The model under review builds one solid part; all positions refer to its coordinate system, in mm. A direction names the side the tool comes from. Give positions to 0.01 mm unless a question says otherwise; leave off trailing zeros. Order: outer loops, then holes, each group sorted by start corner. A loop starts at its lowest first (then second) coordinate and runs counter-clockwise, first axis right, second up. Notation, with made-up numbers: M 40,23 L 70,23 A19 cw 70,50 Z; hole C -32,22 d1. An arc over 180 degrees is marked long. One line per question, with ' | ' between items. Start each with the question number.
1. We need section C-C on z = 2.5. Write out the cut boundary in (x, y), then the cut area to 3 significant figures.
2. The part is to be moulded in two halves that separate along X. For faces 1 (the face through (-24.927, -8, -1)), 2 (the face through (-12.3, -0.6, 6.5)), 3 (the face through (-24.4, -6.1, 7.404)), say which applies: +X half, -X half, draft (parallel to the pull), parting line (faces both ways), or undercut.
3. Insertion check: P1, Ø8.5, axis at x = -15.4, z = -6.46, coming from the +Y side; P2, Ø5, axis at y = -6, z = 2, coming from the -X side; P3, Ø8, axis at x = 8.5, z = -2, coming from the -Y side; P4, Ø1.1, axis at x = 25.5, y = -8, coming from the -Z side. Each pin has a flat end and moves straight along its axis. Give the tip position at first contact, or say it passes through.
4. Wall thickness on L1, parallel to Z at x = 0, y = -0.95; L2, parallel to X at y = -9, z = -9; L3, parallel to X at y = -0.25, z = -4.75 (3 decimals): over which ranges is each line inside the solid? List them lowest first.
5. For faces 4 (the face through (24.807, -6, -3)), 5 (the face through (25.848, -5, -3)), list the 3-axis set-ups (+Z, -Z, +X, -X, +Y, -Y) from which the entire face can be reached by the end or side of a thin tool; tool diameter is ignored.
6. We need section A-A on y = -2. Write out the cut boundary in (x, z), then the cut area to 3 significant figures.
7. We need section B-B on x = 0. Write out the cut boundary in (y, z).
8. We need section D-D on y = -6.5. Write out the cut boundary in (x, z).
```python
from build123d import *

# Parameters (mm, degrees)
F0_W     = 50.8
F0_H     = 25.4
F1_DEPTH = 1.27
F3_D     = 6.35
F4_R     = 5.08
F5_W     = 1.0414
F5_H     = 16.51
F6_DEPTH = 10.9728
F7_DEPTH = 0.254
F9_D     = 3.81


with BuildPart() as f1:
    # F0 (on Front) → F1 (new body)
    with BuildSketch(Plane.XZ):
        with Locations((0.432136, -0.480445)):
            Rectangle(F0_W, F0_H)
    extrude(amount=F1_DEPTH)

    # F3 (through all)
    with Locations(Plane.XZ.offset(1.27)):
        with Locations((0, -6.53336), (16.458306, 6.398361), (0, 6.395109), (16.458306, -6.737123), (-15.397238, -6.455945), (-15.474654, 6.395109)):
            Hole(F3_D / 2)

    # F4
    f4_edges = [f1.edges().sort_by_distance(p)[0] for p in [
        (25.832136, -0.635, 12.219555),
        (25.832136, -0.635, -13.180445),
        (-24.967864, -0.635, 12.219555),
        (-24.967864, -0.635, -13.180445),
    ]]
    fillet(f4_edges, radius=F4_R)

    # F5 (on Front) → F6 (join)
    with BuildSketch(Plane.XZ):
        with Locations((25.327766, -0.851475)):
            Rectangle(F5_W, F5_H)
        with Locations((-24.406663, -0.851475)):
            Rectangle(F5_W, F5_H)
    extrude(amount=F6_DEPTH)

    # F5 (on Front) → F7 (join)
    with BuildSketch(Plane.XZ):
        with Locations((25.327766, -0.851475)):
            Rectangle(F5_W, F5_H)
        with Locations((-24.406663, -0.851475)):
            Rectangle(F5_W, F5_H)
    extrude(amount=F7_DEPTH)

    # F9 (through all)
    with Locations(Plane.YZ.offset(25.848466)):
        with Locations((-5.532465, -0.73287)):
            Hole(F9_D / 2)


solid = f1.part
```
Entries:
1) outline: M -24.97,-1.27 L -24.93,-1.27 L -24.93,-10.97 L -23.89,-10.97 L -23.89,-1.27 L 24.81,-1.27 L 24.81,-10.97 L 25.85,-10.97 L 25.85,0 L -24.97,0 Z | area: 84.7 mm^2
2) face 1: -X half | face 2: undercut | face 3: draft
3) P1: stops at y = 0 | P2: stops at x = -24.93 | P3: stops at y = -1.27 | P4: stops at z = -9.11
4) L1: z = -13.18 to -9.71, -3.36 to 3.22, 9.57 to 12.22 | L2: x = -24.93 to -23.89, 24.81 to 25.85 | L3: x = -24.968 to -18.075, -12.719 to -2.627, 2.627 to 13.982, 18.935 to 25.848
5) face 4: +Z, -Z, -Y | face 5: +Z, -Z, +X, +Y, -Y
6) outline: M -24.93,-9.11 L -23.89,-9.11 L -23.89,7.4 L -24.93,7.4 Z; M 24.81,-9.11 L 25.85,-9.11 L 25.85,7.4 L 24.81,7.4 Z | area: 34.4 mm^2
7) outline: M -1.27,-13.18 L 0,-13.18 L 0,-9.71 L -1.27,-9.71 Z; M -1.27,-3.36 L 0,-3.36 L 0,3.22 L -1.27,3.22 Z; M -1.27,9.57 L 0,9.57 L 0,12.22 L -1.27,12.22 Z
8) outline: M -24.93,-9.11 L -23.89,-9.11 L -23.89,-2.37 L -24.93,-2.37 Z; M -24.93,0.91 L -23.89,0.91 L -23.89,7.4 L -24.93,7.4 Z; M 24.81,-9.11 L 25.85,-9.11 L 25.85,-2.37 L 24.81,-2.37 Z; M 24.81,0.91 L 25.85,0.91 L 25.85,7.4 L 24.81,7.4 Z
